Verification items for this drawing (mm, ordinates from the low corner). A direction names the side the tool comes from. Round coordinates to 2 decimals unless told otherwise and drop trailing zeros. Order: outer loops, then holes, each group sorted by start corner. A loop starts at its lowest first (then second) coordinate and runs counter-clockwise, first axis right, second up. Notation, with made-up numbers: M -27.5,5 L 1.5,5 A15 cw 1.5,21 Z; hole C -30,23 d11. An arc over 180 degrees is marked long. Return JSON: item names as keys, results as strings. Group by question number.
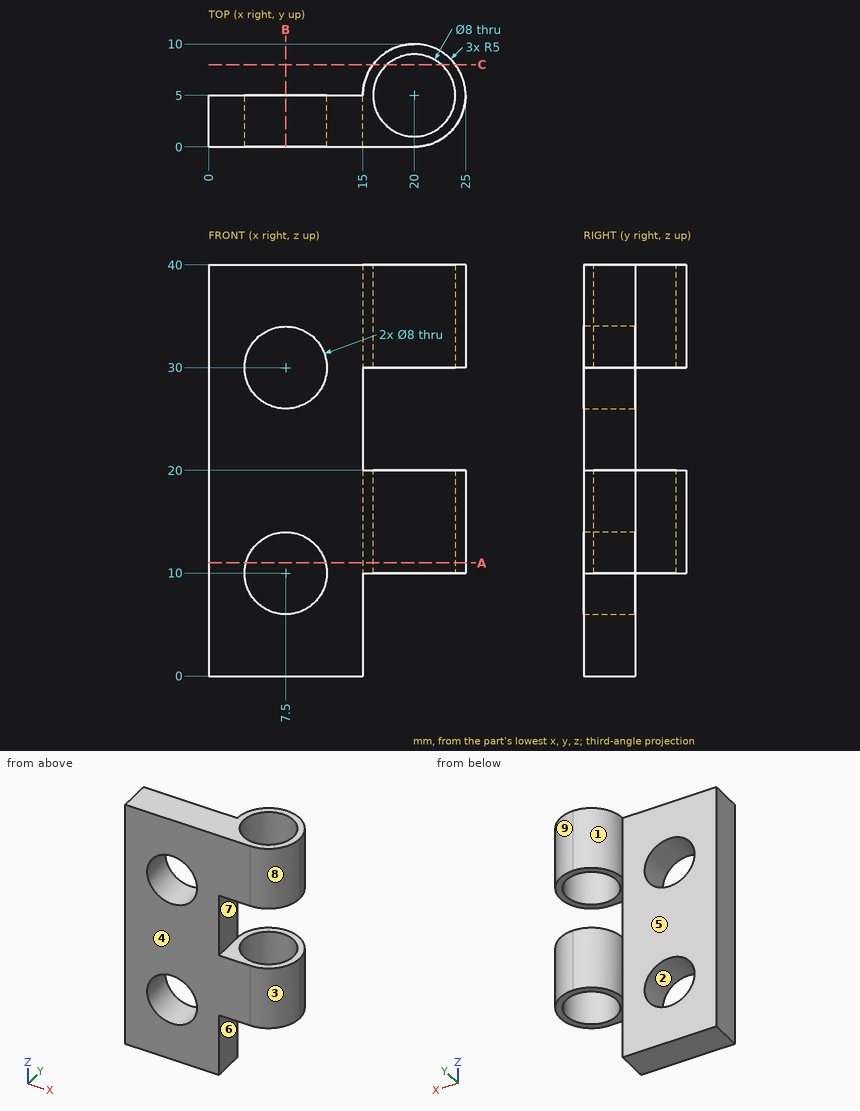
Q1. Depth check by flat-ended pin: pin 1 Ø5 at (x, y) = (20.5, 3) entering from -Z; pin 2 Ø5.5 at (y, z) = (2, 23.5) entering from +X; pin 3 Ø1 at (y, z) = (6, 16.5) entering from -X (3 decimals); pin 4 Ø3 at (x, y) = (20.5, 3.5) entering from +Z. Enter the tip coordinate at first touch or a pass-through.
Q2. Material ranges on line 1 along Z through (x, y) = (15.25, 5.5); line 2 along Z through (x, y) = (4, 2.25); line 3 along Y through (x, z) = (20, 36.5), recorded low to high.
Q3. Section check B-B on x = 7.5. Record the cut outline in (y, z).
Q4. Section check A-A on z = 11. Count the separate pieces of the cut face and the enclosed holes in it, plus the area to 3 significant figures.
Q5. Set-up check for the marked faces 5, 6, 7, 8 and 9: record each of +Z, -Z, +X, -X, +Y, -Y from which the full face is reachable in a straight line by a thin tool's end or side.
Q6. Section check C-C on y = 8. Record the cut outline in (x, z).
Q7. Release check for a two-part mould opening along X. For the marked faces 1, 2, 3 and 4 record: +X half, -X half, draft (parallel to the pull), parting line (faces both ways), or undercut.
Geometry check:
{
 "1": {"pin 1": "stops at z = 10", "pin 2": "stops at x = 15", "pin 3": "stops at x = 15.025", "pin 4": "passes through"},
 "2": {"line 1": "z = 10 to 20, 30 to 40", "line 2": "z = 0 to 8.06, 11.94 to 28.06, 31.94 to 40", "line 3": "y = 0 to 1, 9 to 10"},
 "3": {"outline": "M 0,0 L 5,0 L 5,6 L 0,6 Z; M 0,14 L 5,14 L 5,26 L 0,26 Z; M 0,34 L 5,34 L 5,40 L 0,40 Z"},
 "4": {"separate pieces": "2", "enclosed holes": "1", "area": "69.9 mm^2"},
 "5": {"face 5": "+Z, -Z, -X, +Y", "face 6": "-Z, +X, +Y, -Y", "face 7": "+X, +Y, -Y", "face 8": "+Z, -Z, +X, -Y", "face 9": "+Z, -Z, +X, +Y"},
 "6": {"outline": "M 16,10 L 17.35,10 L 17.35,20 L 16,20 Z; M 16,30 L 17.35,30 L 17.35,40 L 16,40 Z; M 22.65,10 L 24,10 L 24,20 L 22.65,20 Z; M 22.65,30 L 24,30 L 24,40 L 22.65,40 Z"},
 "7": {"face 1": "-X half", "face 2": "undercut", "face 3": "+X half", "face 4": "draft"}
}
